from build123d import *

# Parameters (mm, degrees)
SKETCH2_W           = 24.765
SKETCH2_H           = 15.875
BOSS_EXTRUDE1_DEPTH = 19.05
SKETCH3_W           = 28.575
SKETCH3_H           = 22.86
BOSS_EXTRUDE2_DEPTH = 38.1
SKETCH4_W           = 6.35
SKETCH4_H           = 23.8125
SKETCH4_W_2         = 11.049
CUT_EXTRUDE1_DEPTH  = 47.6725
FILLET5_R           = 11.43
SKETCH7_R           = 6.477
CUT_EXTRUDE3_DEPTH  = 46.56539833
FILLET3_R           = 6.35
CHAMFER1_SIZE       = 5.08


with BuildPart() as part:
    # Sketch2 → Boss-Extrude1 (new body)
    with BuildSketch(Plane.XY):
        Rectangle(SKETCH2_W, SKETCH2_H)
    extrude(amount=-BOSS_EXTRUDE1_DEPTH)

    # Sketch3 → Boss-Extrude2 (add)
    with BuildSketch(Plane.XY):
        Rectangle(SKETCH3_W, SKETCH3_H)
    extrude(amount=BOSS_EXTRUDE2_DEPTH)

    # Sketch4 → Cut-Extrude1 (cut, through all)
    with BuildSketch(Plane(origin=(0, -11.43, 0), x_dir=(-1, 0, 0), z_dir=(0, -1, 0))):
        with Locations((11.1125, -26.19375)):
            Rectangle(SKETCH4_W, SKETCH4_H)
        with Locations((-3.175, -26.19375)):
            Rectangle(SKETCH4_W_2, SKETCH4_H)
    extrude(amount=-CUT_EXTRUDE1_DEPTH, mode=Mode.SUBTRACT)

    # Fillet5
    fillet5_edges = [part.edges().sort_by_distance(p)[0] for p in [
        (-5.1435, -11.43, 38.1),
        (-5.1435, 11.43, 38.1),
        (11.4935, 11.43, 38.1),
        (11.4935, -11.43, 38.1),
    ]]
    fillet(fillet5_edges, radius=FILLET5_R - 0.0001)  # a hair under: the kernel refuses the full size

    # Sketch7 → Cut-Extrude3 (cut, through all)
    with BuildSketch(Plane.ZY.offset(7.9375)):
        with Locations(Location((26.67, 0, 0), (0, 0, 270))):
            Circle(SKETCH7_R)
    extrude(amount=-CUT_EXTRUDE3_DEPTH, mode=Mode.SUBTRACT)

    # Fillet3
    fillet3_edges = [part.edges().sort_by_distance(p)[0] for p in [
        (-12.3825, 7.9375, -9.525),
        (12.3825, 7.9375, -9.525),
        (12.3825, -7.9375, -9.525),
        (-12.3825, -7.9375, -9.525),
    ]]
    fillet(fillet3_edges, radius=FILLET3_R)

    # Chamfer1
    chamfer1_edges = [part.edges().sort_by_distance(p)[0] for p in [
        (-11.1125, 11.43, 14.2875),
        (-11.1125, -11.43, 14.2875),
        (3.175, 11.43, 14.2875),
        (3.175, -11.43, 14.2875),
    ]]
    chamfer(chamfer1_edges, length=CHAMFER1_SIZE)


solid = part.part
Source: CAD feature listing. Evaluate the final solid. Frame: model axes, mm. A direction names the side the tool comes from. Give positions to 0.01 mm unless a question says otherwise; leave off trailing zeros. Loops run counter-clockwise (first coordinate to the right, second up) from the corner with the lowest first, then second, coordinate; pieces in that order, holes last. Notation, with made-up numbers: (9.25, 4.5) -> (37.25, 4.5) arc R26 cw to (37.25, 39.5) -> close; hole circle Ø6 at (10.25, 50.25). An arc over 180 degrees is marked (long way). Use a Markdown table: item, result. Add a question column.
1) Section query D-D, the plane z = 26. Return the cut outline in (x, y), then the cut area to 3 significant figures.
2) Line query: line 1 along Y through (x, z) = (-7.5, 26.5); line 2 along Z through (x, y) = (-3.95, 0); line 3 along X through (y, z) = (4.5, 32.5). Output: solid intervals per line, ascending. Write a range as [from, to].
3) Reachability of faces 1 (the face through (0, 7.938, -9)), 2 (the face through (10.6, 6, -9.7)), 3 (the face through (3.252, -8.854, 11.783)) from +Z, -Z, +X, -X, +Y, -Y: full face, straight path, thin tool, end or side. Return the list, or none.
4) Section query C-C, the plane z = -5.5. Return the cut outline in (x, y), then the cut area to 3 significant figures.
5) Pull-direction query (X, two-part tool) for faces 4 (the face through (0, -10, 0)), 5 (the face through (-2.35, -2.7, 20.6)), 6 (the face through (-7.938, -2.7, 20.6)); classes: +X half, -X half, draft (parallel to the pull), parting line (faces both ways), or undercut.
6) Section query B-B, the plane y = -0.75. Return the cut outline in (x, z).
7) First-contact query: pin 1 (8 mm diameter, centred on x = -11.5, y = 2, fed in from +Z); pin 2 (1 mm diameter, centred on x = -4.5, y = -3, fed in from +Z); pin 3 (13.5 mm diameter, centred on x = -2.5, z = -8.5, fed in from -Y). Flat tips, straight axial feed; report the tip coordinate or a pass-through.
Numbers:
| question | item | result |
|---|---|---|
| 1 | outline | (-7.94, -11.43) -> (-2.35, -11.43) -> (-2.35, -6.44) -> (-7.94, -6.44) -> close; (-7.94, 6.44) -> (-2.35, 6.44) -> (-2.35, 11.43) -> (-7.94, 11.43) -> close; (8.7, -11.43) -> (14.29, -11.43) -> (14.29, -6.44) -> (8.7, -6.44) -> close; (8.7, 6.44) -> (14.29, 6.44) -> (14.29, 11.43) -> (8.7, 11.43) -> close |
| 1 | area | 111 mm2 |
| 2 | line 1 | y = [-11.43, -6.47], [6.47, 11.43] |
| 2 | line 2 | z = [-19.05, 20.19], [33.15, 38.1] |
| 2 | line 3 | x = [-7.94, -2.35], [8.7, 14.29] |
| 3 | face 1 | -Z, +X, -X, +Y |
| 3 | face 2 | -Z, +X, +Y |
| 3 | face 3 | +Z, -Y |
| 4 | outline | (-12.38, -1.59) arc R6.35 ccw to (-6.03, -7.94) -> (6.03, -7.94) arc R6.35 ccw to (12.38, -1.59) -> (12.38, 1.59) arc R6.35 ccw to (6.03, 7.94) -> (-6.03, 7.94) arc R6.35 ccw to (-12.38, 1.59) -> close |
| 4 | area | 359 mm2 |
| 5 | face 4 | draft |
| 5 | face 5 | undercut |
| 5 | face 6 | -X half |
| 6 | outline | (-14.29, 0) -> (-12.38, 0) -> (-12.38, -19.05) -> (12.38, -19.05) -> (12.38, 0) -> (14.29, 0) -> (14.29, 20.24) -> (8.7, 20.24) -> (8.7, 14.29) -> (-2.35, 14.29) -> (-2.35, 20.24) -> (-7.94, 20.24) -> (-7.94, 14.29) -> (-14.29, 14.29) -> close; (-7.94, 33.1) -> (-2.35, 33.1) -> (-2.35, 38.08) -> (-7.94, 38.08) -> close; (8.7, 33.1) -> (14.29, 33.1) -> (14.29, 38.08) -> (8.7, 38.08) -> close |
| 7 | pin 1 | stops at z = 38.1 |
| 7 | pin 2 | stops at z = 37.82 |
| 7 | pin 3 | stops at y = -7.94 |
